Autodesk Inventor part; units mm, degrees
ref_plane "YZ Plane" through (0, 0, 0) normal (1, 0, 0) x (0, 1, 0)
ref_plane "XZ Plane" through (0, 0, 0) normal (0, 1, 0) x (-1, 0, 0)
ref_plane "XY Plane" through (0, 0, 0) normal (0, 0, 1) x (1, 0, 0)
sketch "Sketch1" plane through (0, 0, 0) normal (0, 1, 0) x (-1, 0, 0)
  circle A0 centre (0, 0) radius 3.275
  circle A1 centre (0, 0) radius 10
  dimension "d0" = 6.55
  dimension "d1" = 20
extrude "Extrusion1" add sketch "Sketch1" along normal blind 8
chamfer "Chamfer1" distance 0.5 angle 45 4 edges at (10, 8, 0) (10, 0, 0) (3.275, 0, 0) (3.275, 8, 0)
sketch "Sketch2" plane through (0, 0, 0) normal (1, 0, 0) x (0, 1, 0)
  circle A0 centre (4, 0) radius 1.425
  line L0 (8, 3.275) -> (8, -3.275)
  line L1 (0, -3.275) -> (0, 3.275)
  line L2 (0, 0) -> (8, 0) construction
  dimension "d7" = 2.85
extrude "Extrusion2" cut sketch "Sketch2" along normal through all both and the other way through all
chamfer "Chamfer2" distance 0.25 angle 45 3 edges at (-9.8979, 4.0001, 1.425) (-9.8979, 4, -1.425) (10, 2.5751, -0.0175)
properties part number "nylonClamp"
Can you work these out from the model? Positions are in its coordinate system, mm. Coordinates: 2 decimals unless noted, no trailing zeros. Loops run counter-clockwise (first coordinate to the right, second up) from the corner with the lowest first, then second, coordinate; pieces in that order, holes last. Notation, with made-up numbers: (75.25, 56.5) -> (90.25, 56.5) arc R32 cw to (90.25, 86.5) -> close; hole circle Ø6 at (-21, -39.75). An arc over 180 degrees is marked (long way). Answer as a JSON object with one key per item and string values.
1) If I drill on line 1 (Z direction, x = 0, y = 4.5) (3 decimals); line 2 (X direction, y = 0.75, z = 2.25); line 3 (Z direction, x = -6.5, y = 4) (3 decimals), over which ranges is the centre line in solid material (lowest first)?
Results:
{"line 1": "z = -10 to -3.275, 3.275 to 10", "line 2": "x = -9.74 to -2.38, 2.38 to 9.74", "line 3": "z = -7.599 to -1.425, 1.425 to 7.599"}
2) For P1, Ø2, axis at x = -7.5, y = 1, coming from the +Z side; P2, Ø1.5, axis at y = 5.5, z = 5, coming from the +X side, each with a flat end and sliding along its axis, tell me the tip position at first contact or that it passes through.
Results:
{"P1": "stops at z = 7.6", "P2": "stops at x = 9.05"}
3) Imagine slicing it at A-A (x = 0). Please give me the cut outline in (y, z) (3 decimals), then the cut area to 3 significant figures.
Results:
{"outline": "(0, -9.5) -> (0.5, -10) -> (7.5, -10) -> (8, -9.5) -> (8, -3.775) -> (7.5, -3.275) -> (0.5, -3.275) -> (0, -3.775) -> close; (0, 3.775) -> (0.5, 3.275) -> (7.5, 3.275) -> (8, 3.775) -> (8, 9.5) -> (7.5, 10) -> (0.5, 10) -> (0, 9.5) -> close", "area": "107 mm^2"}
4) Thinking about a two-plate mould opening in Z: for faces 1 (the face through (0, 8, -4)), 2 (the face through (-9.237, 3.951, 3.83)), 3 (the face through (2.6, 3.95, 1.99)), which applies, pulls with the +Z half, pulls with the -Z half, needs draft (parallel to the pull), parting line crosses it, or undercut?
Results:
{"face 1": "needs draft", "face 2": "parting line crosses it", "face 3": "undercut"}
5) Imagine slicing it at B-B (y = 6.75). Please give me the cut outline in (x, z) (3 decimals).
Results:
{"outline": "circle Ø20 at (0, 0); hole circle Ø6.55 at (0, 0)"}
